Geometry: final body of the model. Coordinates: model frame, mm. Face numbers are marked on the shaded views. A direction names the side the tool comes from. Round coordinates to 2 decimals unless told otherwise and drop trailing zeros. Write each loop counter-clockwise with the first axis right and the second up, starting at its lowest first coordinate (ties: lowest second). Pieces come first, ordered by that corner, then holes. Notation, with made-up numbers: (30.5, 28) -> (37.5, 28) arc R8 cw to (37.5, 42) -> close; hole circle Ø6 at (-37, -30.75). An arc over 180 degrees is marked (long way). Use one line per item in the form item = value. Start each with the question number.
1. Reachability of the marked faces 1 and 2 from +Z, -Z, +X, -X, +Y, -Y: full face, straight path, thin tool, end or side. Return the list, or none.
2. Line query: L1, parallel to Z at x = 10, y = 2; L2, parallel to X at y = 2.5, z = -12.75; L3, parallel to Y at x = -3.3, z = 0. Output: solid intervals per line, ascending.
3. Cut plane B-B, the plane y = 4.5. Return the cut outline in (x, z).
4. Pin query (flat end, axial travel): pin 1 Ø8 at (x, z) = (-10.5, -6) entering from -Y; pin 2 Ø1 at (x, z) = (-6.5, 8) entering from +Y (3 decimals); pin 3 Ø1 at (x, y) = (5, -3) entering from +Z. Return the tip coordinate at first contact, or that it passes through.
5. Cut plane A-A, the plane y = -3. Return the cut outline in (x, z), plus the area to 3 significant figures.
6. Cut plane C-C, the plane x = 10.5. State how many separate pieces and enclosed holes the cut face has, plus the area to 3 significant figures.
7. Draft query along Z for the marked faces 3, 4 and 5. Return one class per face: pulls with the +Z half, pulls with the -Z half, needs draft (parallel to the pull), parting line crosses it, or undercut.
```python
from build123d import *

# Parameters (mm, degrees)
EXTRUDE_1_DEPTH                         = 5
SKETCH_3_R                              = 5.5
EXTRUDE_2_DEPTH                         = 5
CUT_EXTRUDE_1083_REACH                  = 23.692
CUT_EXTRUDE_1083_END_RADIUS             = 5.5
SKETCH_6_R                              = 1.5
CUT_EXTRUDE_1083_DIRECTION_2_REACH      = 23.692
CUT_EXTRUDE_1083_DIRECTION_2_END_RADIUS = 5.5
FILLET_1_R                              = 0.5
PATTERN_CIRCULAR_1_COUNT                = 6
HOLE_WIZARD_6_0_6_1_D                   = 6
HOLE_WIZARD_6_0_6_1_DEPTH               = 13.5
HOLE_WIZARD_6_0_6_1_TIP                 = 1.802581857


with BuildPart() as part:
    # 草图1 → 凸台-拉伸1 (new body)
    with BuildSketch(Plane(origin=(0, 0, 0), x_dir=(1, 0, 0), z_dir=(0, 1, 0))):
        with BuildLine():
            Line((11.802472048, 9.257518758), (13.918482445, 5.592481242))
            ThreePointArc((13.918482445, 5.592481242), (15, 0), (13.918482445, -5.592481242))
            Line((13.918482445, -5.592481242), (11.802472048, -9.257518758))
            ThreePointArc((11.802472048, -9.257518758), (7.5, -12.990381057), (2.116010397, -14.85))
            Line((2.116010397, -14.85), (-2.116010397, -14.85))
            ThreePointArc((-2.116010397, -14.85), (-7.5, -12.990381057), (-11.802472048, -9.257518758))
            Line((-11.802472048, -9.257518758), (-13.918482445, -5.592481242))
            ThreePointArc((-13.918482445, -5.592481242), (-15, 0), (-13.918482445, 5.592481242))
            Line((-13.918482445, 5.592481242), (-11.802472048, 9.257518758))
            ThreePointArc((-11.802472048, 9.257518758), (-7.5, 12.990381057), (-2.116010397, 14.85))
            Line((-2.116010397, 14.85), (2.116010397, 14.85))
            ThreePointArc((2.116010397, 14.85), (7.5, 12.990381057), (11.802472048, 9.257518758))
        make_face()
    extrude(amount=EXTRUDE_1_DEPTH)

    # 草图3 → 凸台-拉伸2 (add)
    with BuildSketch(Plane.XZ):
        with Locations(Location((0, 0, 0), (0, 0, 90))):
            Circle(SKETCH_3_R)
    extrude(amount=EXTRUDE_2_DEPTH)

    # Cut-Extrude 1083: up to this cylinder (the profile starts inside it)
    cut_extrude_1083_end = Plane(origin=(0, -2.5, 0), z_dir=(0, 1, 0)) * Cylinder(CUT_EXTRUDE_1083_END_RADIUS, 59.384, mode=Mode.PRIVATE)
    # 草图6 → Cut-Extrude 1083 (cut, up to the surface)
    with BuildSketch(Plane(origin=(0, 0, 0), x_dir=(0, 0, -1), z_dir=(1, 0, 0)), mode=Mode.PRIVATE) as cut_extrude_1083_sk1:
        with Locations(Location((0, -2.5, 0), (0, 0, 180))):
            Circle(SKETCH_6_R)
    cut_extrude_1083_tool1 = extrude(cut_extrude_1083_sk1.sketch, amount=-CUT_EXTRUDE_1083_REACH, mode=Mode.PRIVATE) & cut_extrude_1083_end
    add(cut_extrude_1083_tool1.solids().sort_by_distance((0, -2.5, 0))[0], mode=Mode.SUBTRACT)

    # Cut-Extrude 1083 direction 2: up to this cylinder (the profile starts inside it)
    cut_extrude_1083_direction_2_end = Plane(origin=(0, -2.5, 0), z_dir=(0, 1, 0)) * Cylinder(CUT_EXTRUDE_1083_DIRECTION_2_END_RADIUS, 59.384, mode=Mode.PRIVATE)
    # 草图6 → Cut-Extrude 1083 direction 2 (cut, up to the surface)
    with BuildSketch(Plane(origin=(0, 0, 0), x_dir=(0, 0, -1), z_dir=(1, 0, 0)), mode=Mode.PRIVATE) as cut_extrude_1083_direction_2_sk1:
        with Locations(Location((0, -2.5, 0), (0, 0, 180))):
            Circle(SKETCH_6_R)
    cut_extrude_1083_direction_2_tool1 = extrude(cut_extrude_1083_direction_2_sk1.sketch, amount=CUT_EXTRUDE_1083_DIRECTION_2_REACH, mode=Mode.PRIVATE) & cut_extrude_1083_direction_2_end
    add(cut_extrude_1083_direction_2_tool1.solids().sort_by_distance((0, -2.5, 0))[0], mode=Mode.SUBTRACT)

    # 草图7 → 旋转1 (revolve)
    with BuildSketch(Plane.XY):
        with BuildLine():
            Line((0, 11), (0, 5))
            Line((0, 5), (14, 5))
            add(Edge.make_bspline(
                [(0, 11), (5.535231894, 10.848067736), (8.992417741, 9.000576886), (10.444270344, 7.717324106), (14, 5)],
                knots=[0, 0, 0, 0, 0, 1, 1, 1, 1, 1], degree=4))
        make_face()
    revolve(axis=Axis((0, 11, 0), (0, -1, 0)))

    # 圆角1
    fillet_1_edges = [part.edges().sort_by_distance(p)[0] for p in [
        (-14, 5, 0),
    ]]
    fillet(fillet_1_edges, radius=FILLET_1_R)

    # 草图8 → M3 螺纹孔1 (revolve, cut)
    with BuildSketch(Plane(origin=(12.860477246, 2.5, 7.425), x_dir=(0.4999999999999996, 0, -0.8660254037844389), z_dir=(0, 1, 0))):
        Polygon((0, 0), (0, 8.751075774), (1.25, 8), (1.25, 0), align=None)
    hole_wizard_m3_1 = revolve(axis=Axis((18.35973856, 2.5, 10.6), (-0.8660254037844389, 0, -0.49999999999999967)), mode=Mode.SUBTRACT)

    # 阵列(圆周)1: M3 螺纹孔1 ×6 about axis
    pattern_circular_1_axis = Axis((0, 0, 0), (0, 1, 0))
    for i in range(1, PATTERN_CIRCULAR_1_COUNT):
        add(hole_wizard_m3_1.rotate(pattern_circular_1_axis, i * 360 / PATTERN_CIRCULAR_1_COUNT), mode=Mode.SUBTRACT)

    # Ø6.0 (6) 直径孔1
    with Locations(Plane(origin=(0, -5, 0), x_dir=(0, 0, -1), z_dir=(0, -1, 0))):
        with Locations((0, 0)):
            Hole(HOLE_WIZARD_6_0_6_1_D / 2, depth=HOLE_WIZARD_6_0_6_1_DEPTH)
            with Locations((0, 0, -(HOLE_WIZARD_6_0_6_1_DEPTH + HOLE_WIZARD_6_0_6_1_TIP / 2))):  # 118° drill point
                Cone(0, HOLE_WIZARD_6_0_6_1_D / 2, HOLE_WIZARD_6_0_6_1_TIP, mode=Mode.SUBTRACT)


solid = part.part
```
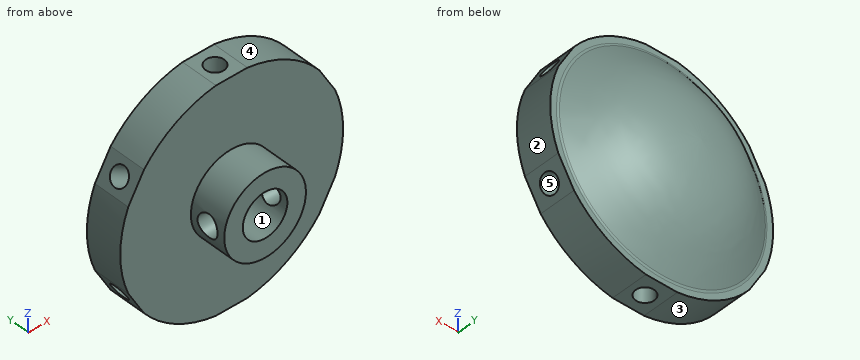
Outcome:
q1.face_1 = -Y
q1.face_2 = +X, +Y, -Y
q2.L1 = -11.18 to -7.1, -4.45 to 4.45, 7.1 to 11.18
q2.L2 = -7.9 to -1.25, 1.25 to 7.9
q2.L3 = -5 to -4, -1 to 10.66
q3.outline = (-13.92, -5.59) -> (-11.8, -9.26) arc R15 ccw to (-2.12, -14.85) -> (2.12, -14.85) arc R15 ccw to (11.8, -9.26) -> (13.92, -5.59) arc R15 ccw to (13.92, 5.59) -> (11.8, 9.26) arc R15 ccw to (2.12, 14.85) -> (-2.12, 14.85) arc R15 ccw to (-11.8, 9.26) -> (-13.92, 5.59) arc R15 ccw to start; hole circle Ø6 at (0, 0)
q4.pin_1 = 0
q4.pin_2 = 8.105
q4.pin_3 = 3.16
q5.outline = (-5.32, -1.41) arc R5.5 ccw to (5.32, -1.41) -> (2.65, -1.41) arc R3 cw to (-2.65, -1.41) -> close; (-5.32, 1.41) -> (-2.65, 1.41) arc R3 cw to (2.65, 1.41) -> (5.32, 1.41) arc R5.5 ccw to start
q5.area = 52.3 mm^2
q6.separate_pieces = 1
q6.enclosed_holes = 2
q6.area = 128 mm^2
q7.face_3 = pulls with the -Z half
q7.face_4 = pulls with the +Z half
q7.face_5 = undercut
